Build history of the part. All positions in model axes, mm. A direction names the side the tool comes from. Coordinates: 2 decimals unless noted, no trailing zeros.
```python
from build123d import *


with BuildPart() as part:
    # Sketch1 → Revolve1 (revolve)
    with BuildSketch(Plane.XY, mode=Mode.PRIVATE) as revolve1_sk:
        with BuildLine():
            Line((0, 0), (-90, 0))
            Line((-90, 0), (-90, 220))
            Line((-90, 220), (-70, 220))
            ThreePointArc((-70, 220), (-60, 210), (-70, 200))
            Line((-70, 200), (-70, 160))
            ThreePointArc((-70, 160), (-50, 140), (-70, 120))
            Line((-70, 120), (-70, 80))
            ThreePointArc((-70, 80), (-45.75081545, 31.814118306), (7.395973154, 22.577181208))
            ThreePointArc((7.395973154, 22.577181208), (11.878862848, 8.608648378), (0, 0))
        make_face()
    revolve(revolve1_sk.sketch.rotate(Axis((-90, 0, 0), (0, 1, 0)), 90), axis=Axis((-90, 0, 0), (0, 1, 0)))


solid = part.part
```
1. 3-axis set-ups, long thin cutter, end or side, ignore diameter. For faces 1 (the face through (-91, 0, 1)), 2 (the face through (-70.476, 179.72, 4.336)): which of +Z, -Z, +X, -X, +Y, -Y reach the whole face in a straight line?
Computed values:
face 1: +Z, -Z, +X, -X, -Y
face 2: none
2. Probe line 1 along Y through (x, z) = (-63, 9); line 2 along Z through (x, y) = (-98.5, 49); line 3 along X through (y, z) = (209.5, -2). List the from-to ranges inside material, lowest first.
Computed values:
line 1: y = 0 to 49.28, 121.88 to 158.12, 204.67 to 215.33
line 2: z = -27.34 to 27.34
line 3: x = -119.92 to -60.08
3. Flat gauge pin, fed straight in: pin 1 (5 mm diameter, centred on x = -114, y = 59.5, fed in from +Z). Where does the tip first touch, or does it go through?
Computed values:
pin 1: stops at z = 10.2
